```python
from build123d import *

# Parameters (mm, degrees)
SKETCH2_W                   = 12.7
SKETCH2_H                   = 22.225
BOSS_EXTRUDE1_DEPTH         = 6.35
BOSS_EXTRUDE1_2_DEPTH       = 6.35
SKETCH2_W_2                 = 19.05
BOSS_EXTRUDE1_3_DEPTH       = 6.35
SKETCH2_3_W                 = 6.35
SKETCH2_3_H                 = 22.225
BOSS_EXTRUDE2_DEPTH         = 31.75
SKETCH3_R                   = 3.175
CUT_EXTRUDE1_DEPTH          = 59.973007597
F_1_4_20_TAPPED_HOLE1_D     = 5.1054
F_1_4_20_TAPPED_HOLE1_DEPTH = 19.05
F_1_4_20_TAPPED_HOLE1_TIP   = 1.533816902
FILLET1_R                   = 8.255


with BuildPart() as part:
    # Sketch2 → Boss-Extrude1 (new body)
    with BuildSketch(Plane(origin=(0, 0, 0), x_dir=(1, 0, 0), z_dir=(0, 1, 0))):
        with Locations((6.35, 11.1125)):
            Rectangle(SKETCH2_W, SKETCH2_H)
    extrude(amount=BOSS_EXTRUDE1_DEPTH)



with BuildPart() as body_2:
    # Sketch2 → Boss-Extrude1 2 (new body)
    with BuildSketch(Plane(origin=(0, 0, 0), x_dir=(1, 0, 0), z_dir=(0, 1, 0))):
        with Locations((50.8, 11.1125)):
            Rectangle(SKETCH2_W, SKETCH2_H)
    extrude(amount=BOSS_EXTRUDE1_2_DEPTH)


with BuildPart() as body_3:
    # Sketch2 → Boss-Extrude1 3 (new body)
    with BuildSketch(Plane(origin=(0, 0, 0), x_dir=(1, 0, 0), z_dir=(0, 1, 0))):
        with Locations((28.575, 11.1125)):
            Rectangle(SKETCH2_W_2, SKETCH2_H)
    extrude(amount=BOSS_EXTRUDE1_3_DEPTH)


with BuildPart() as part_1:
    add(part.part)

    add(body_2.part)  # Boss-Extrude2 merges body 2

    add(body_3.part)  # Boss-Extrude2 merges body 3
    # Sketch2_3 → Boss-Extrude2 (add)
    with BuildSketch(Plane(origin=(0, 0, 0), x_dir=(1, 0, 0), z_dir=(0, 1, 0))):
        with Locations((15.875, 11.1125)):
            Rectangle(SKETCH2_3_W, SKETCH2_3_H)
        with Locations((41.275, 11.1125)):
            Rectangle(SKETCH2_3_W, SKETCH2_3_H)
    extrude(amount=BOSS_EXTRUDE2_DEPTH)

    # Sketch3 → Cut-Extrude1 (cut, through all)
    with BuildSketch(Plane.ZY.offset(-12.7)):
        with Locations(Location((-11.1125, 25.4, 0), (0, 0, 180))):
            Circle(SKETCH3_R)
    extrude(amount=-CUT_EXTRUDE1_DEPTH, mode=Mode.SUBTRACT)

    # 1_4-20 Tapped Hole1
    with Locations(Plane(origin=(6.35, 6.35, -11.1125), x_dir=(0, 0, 1), z_dir=(0, 1, 0))):
        with Locations((0, 0), (0, 22.225), (0, 44.45)):
            Hole(F_1_4_20_TAPPED_HOLE1_D / 2, depth=F_1_4_20_TAPPED_HOLE1_DEPTH)
            with Locations((0, 0, -(F_1_4_20_TAPPED_HOLE1_DEPTH + F_1_4_20_TAPPED_HOLE1_TIP / 2))):  # 118° drill point
                Cone(0, F_1_4_20_TAPPED_HOLE1_D / 2, F_1_4_20_TAPPED_HOLE1_TIP, mode=Mode.SUBTRACT)

    # Fillet1
    fillet1_edges = [part_1.edges().sort_by_distance(p)[0] for p in [
        (15.875, 31.75, -22.225),
        (41.275, 31.75, -22.225),
        (41.275, 31.75, 0),
        (15.875, 31.75, 0),
    ]]
    fillet(fillet1_edges, radius=FILLET1_R)


solid = part_1.part
```
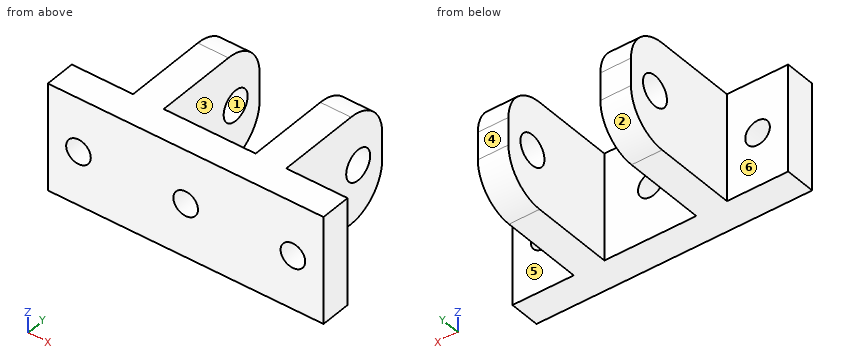
Part model, mm, in its own coordinate system. Face numbers are marked on the shaded views. A direction names the side the tool comes from. Give positions to 0.01 mm unless a question says otherwise; leave off trailing zeros. Order: outer loops, then holes, each group sorted by start corner. A loop starts at its lowest first (then second) coordinate and runs counter-clockwise, first axis right, second up. Notation, with made-up numbers: M 64.25,24.5 L 99.25,24.5 A12 ccw 99.25,42.5 Z; hole C 65.25,-39 d5. An arc over 180 degrees is marked long. Use a Markdown table: item, result. Add a question column.
(1) Saw through at B-B, the plane x = 50.8. Give the cut face in (y, z) (3 decimals).
(2) Saw through at D-D, the plane y = 27.5. Give the cut face in (x, z), and give its area (3 significant figures).
(3) Probe line 1 along X through (y, z) = (9.5, -3); line 2 along Y through (x, z) = (22, -8); line 3 along Y through (x, z) = (15, -10.25). List the from-to ranges inside material, lowest first. Write a range as [from, to].
(4) Saw through at A-A, the plane y = 12.5. Give the cut face in (x, z) (3 decimals), and give its area (3 significant figures).
(5) Saw through at C-C, the plane z = -12.5. Give the number of separate pieces and of enclosed holes in the cut face, and give its area (3 significant figures).
(6) 3-axis set-ups, long thin cutter, end or side, ignore diameter. For the marked faces 4, 5 and 6: which of +Z, -Z, +X, -X, +Y, -Y reach the whole face in a straight line?
(7) Mould opens along Y. For the marked faces 1, 2 and 3 say: +Y half, -Y half, draft (parallel to the pull), parting line (faces both ways), or undercut.
(8) Drop flat-ended pins along their axis: P1, Ø10, axis at x = 10.5, z = -15, coming from the +Y side; P2, Ø2, axis at x = 34, z = -10, coming from the +Y side; P3, Ø3, axis at y = 11.5, z = -10, coming from the -X side; P4, Ø8.5, axis at y = 25.4, z = -11.11, coming from the +X side. Give the stop position or say it passes through.
Answer key:
| question | item | result |
|---|---|---|
| 1 | outline | M 0,-22.225 L 6.35,-22.225 L 6.35,-13.665 L 0,-13.665 Z; M 0,-8.56 L 6.35,-8.56 L 6.35,0 L 0,0 Z |
| 2 | outline | M 12.7,-21.19 L 19.05,-21.19 L 19.05,-13.49 L 12.7,-13.49 Z; M 12.7,-8.73 L 19.05,-8.73 L 19.05,-1.04 L 12.7,-1.04 Z; M 38.1,-21.19 L 44.45,-21.19 L 44.45,-13.49 L 38.1,-13.49 Z; M 38.1,-8.73 L 44.45,-8.73 L 44.45,-1.04 L 38.1,-1.04 Z |
| 2 | area | 195 mm^2 |
| 3 | line 1 | [12.7, 19.05], [38.1, 44.45] |
| 3 | line 2 | [0, 6.35] |
| 3 | line 3 | [0, 22.34], [28.46, 31.75] |
| 4 | outline | M 12.7,-22.225 L 19.05,-22.225 L 19.05,0 L 12.7,0 Z; M 38.1,-22.225 L 44.45,-22.225 L 44.45,0 L 38.1,0 Z |
| 4 | area | 282 mm^2 |
| 5 | separate pieces | 6 |
| 5 | enclosed holes | 0 |
| 5 | area | 531 mm^2 |
| 6 | face 4 | +Z, -Z, +X, -X, +Y |
| 6 | face 5 | +Z, -Z, +X, +Y |
| 6 | face 6 | +Z, -Z, -X, +Y |
| 7 | face 1 | undercut |
| 7 | face 2 | +Y half |
| 7 | face 3 | draft |
| 8 | P1 | y = 31.75 |
| 8 | P2 | y = 6.35 |
| 8 | P3 | x = 12.7 |
| 8 | P4 | x = 44.45 |
